Geometry: final body of the model. Coordinates: model frame, mm. Face numbers are marked on the shaded views. A direction names the side the tool comes from. Give positions to 0.01 mm unless a question says otherwise; leave off trailing zeros. Order: outer loops, then holes, each group sorted by start corner. A loop starts at its lowest first (then second) coordinate and runs counter-clockwise, first axis right, second up. Notation, with made-up numbers: (33, 29.25) -> (55, 29.25) arc R28 cw to (55, 60.25) -> close; hole circle Ø1 at (24, 13.5). An arc over 180 degrees is marked (long way). One line per question, with ' | ' between items. Start each with the question number.
(1) Section A-A (y = -13.25). State how many separate pieces and enclosed holes the cut face has, then the cut area to 3 significant figures.
(2) First-contact query: pin 1 Ø6 at (y, z) = (-11.5, 49.5) entering from -X; pin 2 Ø1 at (x, y) = (25.5, -13.5) entering from -Z; pin 3 Ø6 at (x, z) = (0, 0) entering from +Y; pin 4 Ø6 at (x, y) = (44, -11) entering from +Z. Flat tips, straight axial feed; report the tip coordinate or a pass-through.
(3) Set-up query: the marked faces 4, 5 and 6. Return all of +Z, -Z, +X, -X, +Y, -Y with unobstructed straight access to the full face (end or side cutting, diameter ignored); none if empty.
(4) Section B-B (x = -7.5). Return loops of the section in (y, z).
(5) Mould query, pull axis Z, two halves, no side actions, for the marked faces 1, 2 and 3. Classes: +Z half, -Z half, draft (parallel to the pull), parting line (faces both ways), or undercut.
(6) Ray query, L1, parallel to Z at x = 44.45, y = -18.25; L2, parallel to Z at x = 2, y = -9; L3, parallel to X at y = -5, z = 0.5. Return the intervals inside material, ascending.
(7) Section C-C (x = 24). Return loops of the section in (y, z), then the cut area to 3 significant figures.
```python
from build123d import *

# Parameters (mm, degrees)
F1_DEPTH = 25.4


with BuildPart() as f1:
    # F0 (on Front) → F1 (new body)
    with BuildSketch(Plane.XZ):
        with BuildLine():
            Line((-9.0993962158, -3.1143001494), (-9.5157433692, 1.3958886217))
            ThreePointArc((-9.5157433692, 1.3958886217), (-9.5768630631, -0.8840649199), (-9.0993962158, -3.1143001494))
        make_face()
        with BuildLine():
            ThreePointArc((0, -9.6175816561), (0.6447692536, -9.5959444309), (1.2866373584, -9.5311301124))
            Line((1.2866373584, -9.5311301124), (0, -9.6175816561))
        make_face()
        with BuildLine():
            ThreePointArc((44.8987295624, 7.924805867), (44.45, 7.9375), (44.0012704376, 7.924805867))
            Line((44.0012704376, 7.924805867), (44.8987295624, 7.924805867))
        make_face()
        with BuildLine():
            Line((15.6009559029, 66.4369712147), (15.8431126272, 64.5056874674))
            ThreePointArc((15.8431126272, 64.5056874674), (15.7516610445, 65.4750441364), (15.6009559029, 66.4369712147))
        make_face()
        with BuildLine():
            ThreePointArc((-14.535897452, 69.8814818237), (-15.7772599915, 65.2588894677), (-15.5843994353, 60.4764062373))
            Line((-15.5843994353, 60.4764062373), (-14.535897452, 69.8814818237))
        make_face()
        with BuildLine():
            ThreePointArc((-9.5157433692, 1.3958886217), (-6.2877978701, 7.2774634906), (0, 9.6175816561))
            Line((0, 9.6175816561), (0, 47.625))
            ThreePointArc((0, 47.625), (-8.849704349, 50.3205327143), (-14.6940962464, 57.4917423074))
            Line((-14.6940962464, 57.4917423074), (-9.5157433692, 1.3958886217))
        make_face()
        with BuildLine():
            ThreePointArc((-14.535897452, 69.8814818237), (-8.6807142865, 76.7913815864), (0, 79.375))
            Line((0, 79.375), (0, 104.775))
            ThreePointArc((0, 104.775), (-7.0993647554, 107.9498310991), (-9.4660714511, 115.357882925))
            Line((-9.4660714511, 115.357882925), (-14.535897452, 69.8814818237))
        make_face()
        with BuildLine():
            Line((0, 104.775), (0, 79.375))
            ThreePointArc((0, 79.375), (10.1338839289, 75.7196571767), (15.6009559029, 66.4369712147))
            Line((15.6009559029, 66.4369712147), (9.4509966267, 115.4850264818))
            ThreePointArc((9.4509966267, 115.4850264818), (9.5064811542, 114.8936674705), (9.525, 114.3))
            ThreePointArc((9.525, 114.3), (6.7351920908, 107.5648079092), (0, 104.775))
        make_face()
        with BuildLine():
            Line((36.5125, 0), (9.6175816561, 0))
            ThreePointArc((9.6175816561, 0), (7.2412780905, -6.3294366675), (1.2866373584, -9.5311301124))
            Line((1.2866373584, -9.5311301124), (40.5179037022, -6.8951087704))
            ThreePointArc((40.5179037022, -6.8951087704), (37.5865125259, -3.9870347306), (36.5125, 0))
        make_face()
        with BuildLine():
            ThreePointArc((9.4509966267, 115.4850264818), (-0.064017057, 123.8247848698), (-9.4660714511, 115.357882925))
            ThreePointArc((-9.4660714511, 115.357882925), (-7.0993647554, 107.9498310991), (0, 104.775))
            ThreePointArc((0, 104.775), (6.7351920908, 107.5648079092), (9.525, 114.3))
            ThreePointArc((9.525, 114.3), (9.5064811542, 114.8936674705), (9.4509966267, 115.4850264818))
        make_face()
        with BuildLine():
            ThreePointArc((3.8802388174, 114.3), (2.7437431804, 111.5562568196), (0, 110.4197611826))
            ThreePointArc((0, 110.4197611826), (-2.7437431804, 117.0437431804), (3.8802388174, 114.3))
        make_face(mode=Mode.SUBTRACT)
        with BuildLine():
            ThreePointArc((44.0012704376, 7.924805867), (38.680871073, 5.4517022731), (36.5125, 0))
            ThreePointArc((36.5125, 0), (37.5865125259, -3.9870347306), (40.5179037022, -6.8951087704))
            ThreePointArc((40.5179037022, -6.8951087704), (48.4370347306, -6.8634874741), (52.3875, 0))
            ThreePointArc((52.3875, 0), (50.219128927, 5.4517022731), (44.8987295624, 7.924805867))
            Line((44.8987295624, 7.924805867), (44.0012704376, 7.924805867))
        make_face()
        with BuildLine():
            ThreePointArc((47.3139224762, 0), (44.45, -2.8639224762), (41.5860775238, 0))
            ThreePointArc((41.5860775238, 0), (44.45, 2.8639224762), (47.3139224762, 0))
        make_face(mode=Mode.SUBTRACT)
        with BuildLine():
            Line((0, 58.5082662054), (0, 47.625))
            ThreePointArc((0, 47.625), (10.1067179605, 51.2578646852), (15.5877554471, 60.4937556452))
            ThreePointArc((15.5877554471, 60.4937556452), (15.8030257027, 61.9900319081), (15.875, 63.5))
            ThreePointArc((15.875, 63.5), (15.8670261542, 64.0030964338), (15.8431126272, 64.5056874674))
            Line((15.8431126272, 64.5056874674), (15.6009559029, 66.4369712147))
            ThreePointArc((15.6009559029, 66.4369712147), (10.1338839289, 75.7196571767), (0, 79.375))
            Line((0, 79.375), (0, 68.4917337946))
            ThreePointArc((0, 68.4917337946), (3.5296888161, 67.0296888161), (4.9917337946, 63.5))
            ThreePointArc((4.9917337946, 63.5), (3.5296888161, 59.9703111839), (0, 58.5082662054))
        make_face()
        with BuildLine():
            ThreePointArc((-14.6940962464, 57.4917423074), (-8.849704349, 50.3205327143), (0, 47.625))
            Line((0, 47.625), (0, 58.5082662054))
            ThreePointArc((0, 58.5082662054), (-4.9917337946, 63.5), (0, 68.4917337946))
            Line((0, 68.4917337946), (0, 79.375))
            ThreePointArc((0, 79.375), (-8.6807142865, 76.7913815864), (-14.535897452, 69.8814818237))
            Line((-14.535897452, 69.8814818237), (-15.5843994353, 60.4764062373))
            ThreePointArc((-15.5843994353, 60.4764062373), (-15.2126223867, 58.9621871877), (-14.6940962464, 57.4917423074))
        make_face()
        with BuildLine():
            ThreePointArc((3.8500225809, 0), (-2.7223770747, -2.7223770747), (0, 3.8500225809))
            Line((0, 3.8500225809), (0, 9.6175816561))
            ThreePointArc((0, 9.6175816561), (-6.2877978701, 7.2774634906), (-9.5157433692, 1.3958886217))
            Line((-9.5157433692, 1.3958886217), (-9.0993962158, -3.1143001494))
            ThreePointArc((-9.0993962158, -3.1143001494), (-5.5922196364, -7.8246377839), (0, -9.6175816561))
            Line((0, -9.6175816561), (1.2866373584, -9.5311301124))
            ThreePointArc((1.2866373584, -9.5311301124), (7.2412780905, -6.3294366675), (9.6175816561, 0))
            Line((9.6175816561, 0), (3.8500225809, 0))
        make_face()
        with BuildLine():
            Line((0, 47.625), (0, 9.6175816561))
            ThreePointArc((0, 9.6175816561), (6.8006572076, 6.8006572076), (9.6175816561, 0))
            Line((9.6175816561, 0), (36.5125, 0))
            ThreePointArc((36.5125, 0), (38.680871073, 5.4517022731), (44.0012704376, 7.924805867))
            Line((44.0012704376, 7.924805867), (22.2047249099, 7.924805867))
            ThreePointArc((22.2047249099, 7.924805867), (11.5375167972, 12.9510094978), (8.6223042709, 24.3770143895))
            Line((8.6223042709, 24.3770143895), (15.5877554471, 60.4937556452))
            ThreePointArc((15.5877554471, 60.4937556452), (10.1067179605, 51.2578646852), (0, 47.625))
        make_face()
        with BuildLine():
            Line((0, 9.6175816561), (0, 3.8500225809))
            ThreePointArc((0, 3.8500225809), (2.7223770747, 2.7223770747), (3.8500225809, 0))
            Line((3.8500225809, 0), (9.6175816561, 0))
            ThreePointArc((9.6175816561, 0), (6.8006572076, 6.8006572076), (0, 9.6175816561))
        make_face()
    extrude(amount=F1_DEPTH)


solid = f1.part
```
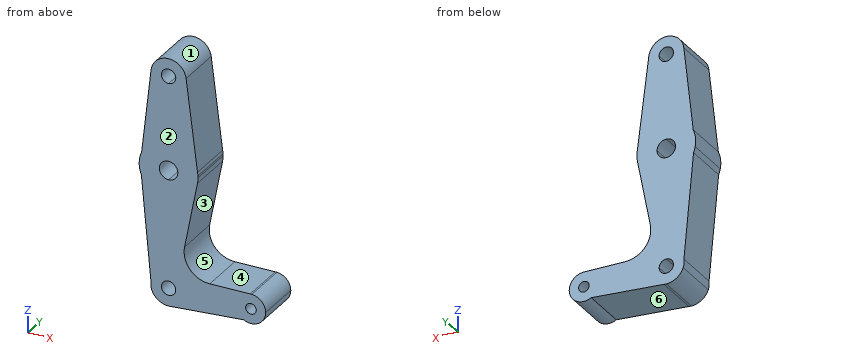
Response:
1) separate pieces: 1 | enclosed holes: 4 | area: 3,570 mm^2
2) pin 1: stops at x = -14.23 | pin 2: stops at z = -7.94 | pin 3: passes through | pin 4: stops at z = 7.94
3) face 4: +Z, +X, +Y, -Y | face 5: +X, +Y, -Y | face 6: -Z, +Y, -Y
4) outline: (-25.4, -6.02) -> (0, -6.02) -> (0, 120.17) -> (-25.4, 120.17) -> close
5) face 1: +Z half | face 2: draft | face 3: undercut
6) L1: z = -7.94 to -2.86, 2.86 to 7.94 | L2: z = -9.48 to -3.29, 3.29 to 58.93, 68.07 to 110.97, 117.63 to 123.61 | L3: x = -9.6 to -3.82, 3.82 to 41.63, 47.27 to 52.37
7) outline: (-25.4, -8) -> (0, -8) -> (0, 7.92) -> (-25.4, 7.92) -> close | area: 405 mm^2
